```python
from build123d import *

# Parameters (mm, degrees)
F1_DEPTH    = 10
F2_DEPTH    = 40
F3_R        = 2.8
F4_DEPTH    = 5
F5_T1_DEPTH = 80.8666856224
F5_T3_DEPTH = 81.0791317508
F6_SIZE     = 5


# Not quite as in the source:
# - a fillet or chamfer that OpenCascade refuses, or shapes differently, is made with other operations: its cross-section is extruded or revolved along the edge and cut away or added


with BuildPart() as f1:
    # F0 (on Top) → F1 (new body)
    with BuildSketch(Plane.XY):
        with BuildLine():
            Line((-43.5517183587, 35.5855710396), (-59.7826302073, -71.725967915))
            Line((-59.7826302073, -71.725967915), (-38.9637436029, -71.725967915))
            Line((-38.9637436029, -71.725967915), (-28.9527400952, -5.5376845384))
            Line((-28.9527400952, -5.5376845384), (-19.966132513, -71.725967915))
            Line((-19.966132513, -71.725967915), (0.2173697927, -71.725967915))
            Line((0.2173697927, -71.725967915), (-14.3378386668, 35.4762497537))
            Line((-14.3378386668, 35.4762497537), (-24.3294449803, 34.076745098))
            ThreePointArc((-24.3294449803, 34.076745098), (-28.9527400952, 27.172764457), (-33.57603521, 34.076745098))
            Line((-33.57603521, 34.076745098), (-43.5517183587, 35.5855710396))
        make_face()
    extrude(amount=F1_DEPTH)

    # F0 (on Top) → F2 (join)
    with BuildSketch(Plane.XY):
        Polygon((-38.9637436029, -71.725967915), (-59.7826302073, -71.725967915), (-59.7826302073, -76.725967915), (0.2173697927, -76.725967915), (0.2173697927, -71.725967915), (-19.966132513, -71.725967915), align=None)
    extrude(amount=F2_DEPTH)

    # F3 (on face) → F4 (cut, through all)
    with BuildSketch(Plane(origin=(0, -71.725967915, 0), x_dir=(-1, 0, 0), z_dir=(0, 1, 0))):
        with Locations((39.7826302073, 25)):
            Circle(F3_R)
        with Locations((19.7826302073, 25)):
            Circle(F3_R)
    extrude(amount=-F4_DEPTH, mode=Mode.SUBTRACT)

    # F5: fillet of radius 15 on 2 edges, made by hand

    # F5_s2 → F5_t1 (cut)
    with BuildSketch(Plane.XY.offset(-35.4333428112)):
        with BuildLine():
            ThreePointArc((-33.57603521, 34.076745098), (-41.6218227772, 29.7568391026), (-45.6713333114, 21.5716237836))
            Line((-45.6713333114, 21.5716237836), (-43.5517183587, 35.5855710396))
            Line((-43.5517183587, 35.5855710396), (-33.57603521, 34.076745098))
        make_face()
    extrude(amount=F5_T1_DEPTH, mode=Mode.SUBTRACT)

    # F5_s4 → F5_t3 (cut)
    with BuildSketch(Plane.XY.offset(-35.5395658754)):
        with BuildLine():
            ThreePointArc((-12.4252559054, 21.3896694023), (-16.3501492828, 29.6353150708), (-24.3294449803, 34.076745098))
            Line((-24.3294449803, 34.076745098), (-14.3378386668, 35.4762497537))
            Line((-14.3378386668, 35.4762497537), (-12.4252559054, 21.3896694023))
        make_face()
    extrude(amount=F5_T3_DEPTH, mode=Mode.SUBTRACT)

    # F6
    f6_edges = [f1.edges().sort_by_distance(p)[0] for p in [
        (0.21737, -74.225968, 40),
        (-59.78263, -74.225968, 40),
    ]]
    chamfer(f6_edges, length=F6_SIZE)


solid = f1.part
```
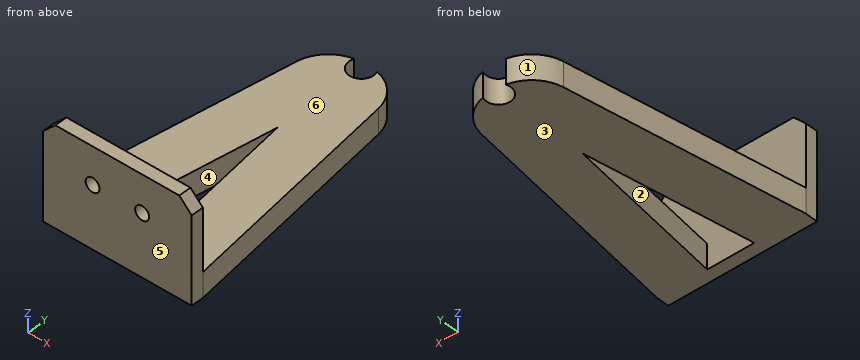
Design review of the part built by this model. Coordinates are the model's own, in mm. Face numbers are marked on the shaded views. A direction names the side the tool comes from. Give positions to 0.01 mm unless a question says otherwise; leave off trailing zeros. Write each loop counter-clockwise with the first axis right and the second up, starting at its lowest first coordinate (ties: lowest second). Pieces come first, ordered by that corner, then holes.
(1) Mouldability with a two-part tool opening along Y and no side actions: class the marked faces 1, 2 and 3 as +Y half, -Y half, draft (parallel to the pull), parting line (faces both ways), or undercut.
Checked values:
face 1: +Y half
face 2: undercut
face 3: draft
(2) Tool access review of the marked faces 4, 5 and 6: name each direction out of +Z, -Z, +X, -X, +Y, -Y from which nothing blocks a thin tool from reaching the whole face with its end or side.
Checked values:
face 4: +Z, -Z
face 5: +Z, -Z, +X, -X, -Y
face 6: +Z, +X, -X, +Y
(3) Add section A-A (z = 25). Give the boundary of the cut face in (x, y).
Checked values:
outline: (-59.78, -76.73) - (-42.58, -76.73) - (-42.58, -71.73) - (-59.78, -71.73) - close; (-36.98, -76.73) - (-22.58, -76.73) - (-22.58, -71.73) - (-36.98, -71.73) - close; (-16.98, -76.73) - (0.22, -76.73) - (0.22, -71.73) - (-16.98, -71.73) - close
(4) Add section D-D (x = -6). Give the boundary of the cut face in (y, z).
Checked values:
outline: (-76.73, 0) - (-25.93, 0) - (-25.93, 10) - (-71.73, 10) - (-71.73, 40) - (-76.73, 40) - close
(5) Clearance check with flat-ended pins moving along their axes: pin 1 Ø13 at (x, y) = (-28.95, 32.17) entering from +Z; pin 2 Ø12 at (x, z) = (-7.5, 9) entering from +Y; pin 3 Ø7.5 at (x, z) = (-19.78, 25) entering from +Y. State where each tip first meets the part, or that it passes through.
Checked values:
pin 1: stops at z = 10
pin 2: stops at y = 25.28
pin 3: stops at y = -71.73
(6) Add section C-C (y = -21). Give the boundary of the cut face in (x, z), and give its area (3 significant figures).
Checked values:
outline: (-52.11, 0) - (-31.29, 0) - (-31.29, 10) - (-52.11, 10) - close; (-26.85, 0) - (-6.67, 0) - (-6.67, 10) - (-26.85, 10) - close
area: 410 mm2
(7) Add section B-B (z = 5.5). Give the boundary of the cut face in (x, y), and give its area (3 significant figures).
Checked values:
outline: (-59.78, -76.73) - (0.22, -76.73) - (0.22, -71.73) - (-12.43, 21.39) arc R15 ccw to (-24.33, 34.08) arc R5 cw (long way) to (-33.58, 34.08) arc R15 ccw to (-45.67, 21.57) - (-59.78, -71.73) - close; hole (-38.96, -71.73) - (-19.97, -71.73) - (-28.95, -5.54) - close
area: 4,290 mm2
(8) Wall thickness on line 1 along Z through (x, y) = (-13, -33); line 2 along Y through (x, z) = (-32, 20); line 3 along X through (y, z) = (-37.5, 8): over which ranges is each line inside the solid? List them lowest first.
Checked values:
line 1: z = 0 to 10
line 2: y = -76.73 to -71.73
line 3: x = -54.61 to -33.79, -24.61 to -4.43
